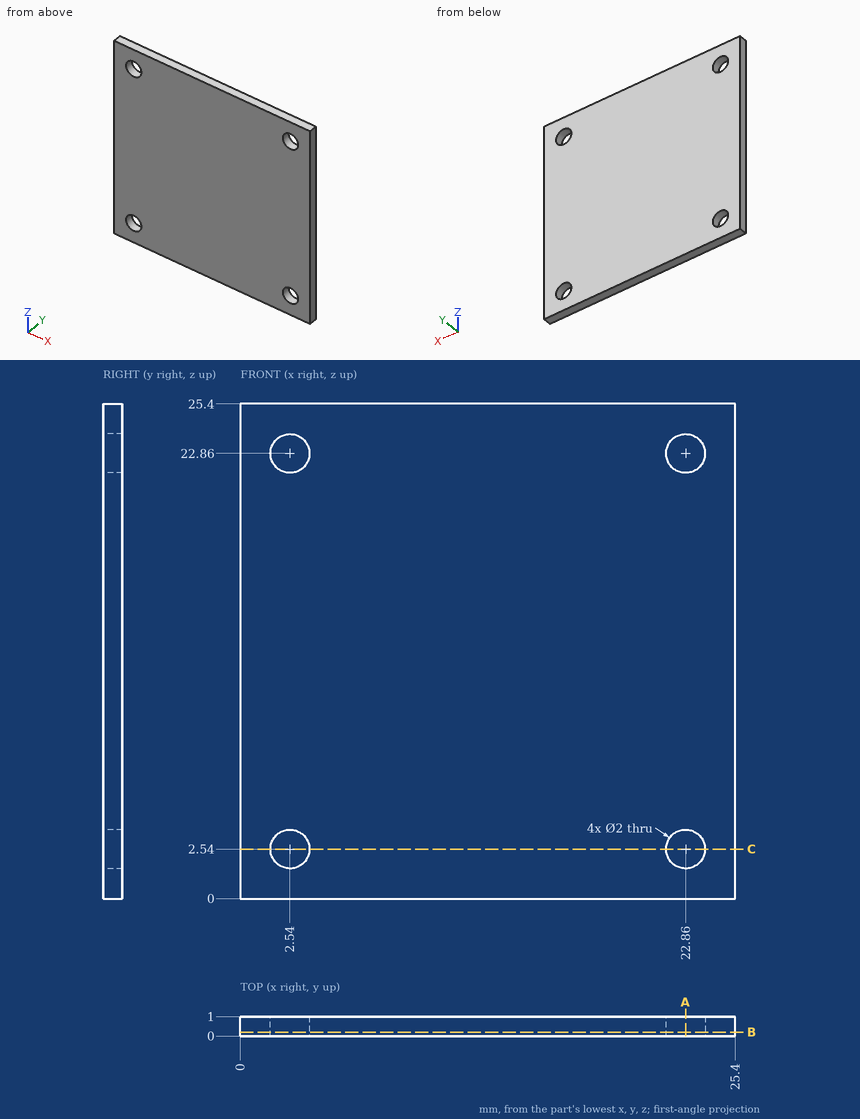
Part print with two shaded views. Sizes in mm from the minimum x, y, z corner. Coordinates: 2 decimals unless noted, no trailing zeros. Loops run counter-clockwise (first coordinate to the right, second up) from the corner with the lowest first, then second, coordinate; pieces in that order, holes last. Notation, with made-up numbers: M 34,35 L 63,35 A21 cw 63,68 Z; hole C 68.25,-23 d2. An arc over 180 degrees is marked long. Use CSV: the item, a comma, the result in double quotes. Start each with the question number.
1. Band-saw the part on B-B, the plane y = 0.2. List the corners of the cut face in (x, z).
2. Band-saw the part on A-A, the plane x = 22.86. List the corners of the cut face in (y, z).
3. Band-saw the part on C-C, the plane z = 2.54. List the corners of the cut face in (x, y).
4. Probe probe 1 along Z at (x, y) = (22.86, 0.3); probe 2 along X at (y, z) = (0.35, 23.75). List the from-to ranges inside material, lowest first. Write a range as [from, to].
Entries:
1,outline,"M 0,0 L 25.4,0 L 25.4,25.4 L 0,25.4 Z; hole C 2.54,2.54 d2; hole C 2.54,22.86 d2; hole C 22.86,2.54 d2; hole C 22.86,22.86 d2"
2,outline,"M 0,0 L 1,0 L 1,1.54 L 0,1.54 Z; M 0,3.54 L 1,3.54 L 1,21.86 L 0,21.86 Z; M 0,23.86 L 1,23.86 L 1,25.4 L 0,25.4 Z"
3,outline,"M 0,0 L 1.54,0 L 1.54,1 L 0,1 Z; M 3.54,0 L 21.86,0 L 21.86,1 L 3.54,1 Z; M 23.86,0 L 25.4,0 L 25.4,1 L 23.86,1 Z"
4,probe 1,"z = [0, 1.54], [3.54, 21.86], [23.86, 25.4]"
4,probe 2,"x = [0, 2.08], [3, 22.4], [23.32, 25.4]"
